Build history of the part. All positions in model axes, mm. Face numbers are marked on the shaded views. Give positions to 0.01 mm unless a question says otherwise; leave off trailing zeros. Loops run counter-clockwise (first coordinate to the right, second up) from the corner with the lowest first, then second, coordinate; pieces in that order, holes last. Notation, with made-up numbers: (61, 71) - (86, 71) arc R14 ccw to (86, 76) - close; hole circle Ø9 at (72.25, 2). An arc over 180 degrees is marked (long way). Return JSON: item names as keys, results as strings. Group by question number.
1) Slice it at D-D (y = 20.75). List the corners of the cut face in (x, z), and give its area (3 significant figures).
2) Drop flat-ended pins along their axis: pin 1 (4 mm diameter, centred on x = 34, z = 0, fed in from +Y); pin 2 (10 mm diameter, centred on x = -30, y = 6.5, fed in from -Z); pin 3 (3 mm diameter, centred on x = 15.5, y = 24, fed in from +Z); pin 4 (18 mm diameter, centred on x = 0, z = 0, fed in from +Y). Give the stop position or say it passes through.
3) Slice it at A-A (x = 0). List the corners of the cut face in (y, z), and give its area (3 significant figures).
4) Drill centre lines: probe 1 along X at (y, z) = (14, 0); probe 2 along Z at (x, y) = (1, 19.5); probe 3 along X at (y, z) = (14, -36.5). Where is each one in solid material? Low to high. Write a range as from..to.
5) Mould opens along X. For the marked faces 1, 2 and 3 say: released by +X, released by -X, zero draft, split by the parting line, or undercut.
6) Slice it at B-B (z = 0). List the corners of the cut face in (x, y).
7) Slice it at C-C (y = 3.75). List the corners of the cut face in (x, z), and give its area (3 significant figures).
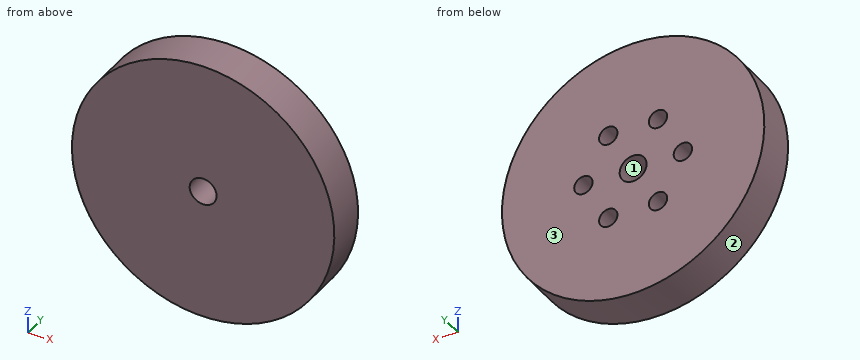
```python
from build123d import *

# Parameters (mm, degrees)
SKETCH1_R             = 97.5
BOSS_EXTRUDE1_DEPTH   = 30
SKETCH2_R             = 10
CUT_EXTRUDE1_DEPTH    = 142.111657917
SKETCH3_R             = 6.819096127
CUT_EXTRUDE2_DEPTH    = 20.141211
CIRPATTERN1_START     = 9.858789147
CIRPATTERN1_OUTLINE_R = 6.819096127
CIRPATTERN1_DEPTH     = 20.141210853


# Read off the part's stored shape, not the designer's step: CirPattern1
with BuildPart() as part:
    # Sketch1 → Boss-Extrude1 (new body)
    with BuildSketch(Plane(origin=(0, 0, 0), x_dir=(1, 0, 0), z_dir=(0, 1, 0))):
        with Locations(Location((0, 0, 0), (0, 0, 270))):
            Circle(SKETCH1_R)
    extrude(amount=BOSS_EXTRUDE1_DEPTH)

    # Sketch2 → Cut-Extrude1 (cut, through all)
    with BuildSketch(Plane(origin=(0, 0, 0), x_dir=(1, 0, 0), z_dir=(0, 1, 0))):
        with Locations(Location((0, 0, 0), (0, 0, 270))):
            Circle(SKETCH2_R)
    extrude(amount=CUT_EXTRUDE1_DEPTH, mode=Mode.SUBTRACT)

    # Sketch3 → Cut-Extrude2 (cut)
    with BuildSketch(Plane(origin=(0, 30, 0), x_dir=(1, 0, 0), z_dir=(0, 1, 0))):
        with Locations(Location((-36.967875527, 0, 0), (0, 0, 270))):
            Circle(SKETCH3_R)
    extrude(amount=-CUT_EXTRUDE2_DEPTH, mode=Mode.SUBTRACT)

    # CirPattern1 outline → CirPattern1 (cut)
    with BuildSketch(Plane(origin=(0, 0, 0), x_dir=(1, 0, 0), z_dir=(0, 1, 0)).offset(CIRPATTERN1_START)):
        with Locations((-18.483937763, -32.01511933)):
            Circle(CIRPATTERN1_OUTLINE_R)
        with Locations((18.483937763, -32.01511933)):
            Circle(CIRPATTERN1_OUTLINE_R)
        with Locations((36.967875527, 0)):
            Circle(CIRPATTERN1_OUTLINE_R)
        with Locations((18.483937763, 32.01511933)):
            Circle(CIRPATTERN1_OUTLINE_R)
        with Locations((-18.483937763, 32.01511933)):
            Circle(CIRPATTERN1_OUTLINE_R)
    extrude(amount=CIRPATTERN1_DEPTH, mode=Mode.SUBTRACT)


solid = part.part
```
Results:
{
 "1": {"outline": "circle Ø195 at (0, 0); hole circle Ø13.64 at (-36.97, 0); hole circle Ø13.64 at (-18.48, -32.02); hole circle Ø13.64 at (-18.48, 32.02); hole circle Ø20 at (0, 0); hole circle Ø13.64 at (18.48, -32.02); hole circle Ø13.64 at (18.48, 32.02); hole circle Ø13.64 at (36.97, 0)", "area": "28,700 mm2"},
 "2": {"pin 1": "y = 9.86", "pin 2": "z = -94.24", "pin 3": "z = 96.49", "pin 4": "through"},
 "3": {"outline": "(0, -97.5) - (30, -97.5) - (30, -10) - (0, -10) - close; (0, 10) - (30, 10) - (30, 97.5) - (0, 97.5) - close", "area": "5,250 mm2"},
 "4": {"probe 1": "-97.5..-43.79, -30.15..-10, 10..30.15, 43.79..97.5", "probe 2": "-97.49..-9.95, 9.95..97.49", "probe 3": "-90.41..-23.62, -13.35..13.35, 23.62..90.41"},
 "5": {"face 1": "undercut", "face 2": "split by the parting line", "face 3": "zero draft"},
 "6": {"outline": "(-97.5, 0) - (-10, 0) - (-10, 30) - (-30.15, 30) - (-30.15, 9.86) - (-43.79, 9.86) - (-43.79, 30) - (-97.5, 30) - close; (10, 0) - (97.5, 0) - (97.5, 30) - (43.79, 30) - (43.79, 9.86) - (30.15, 9.86) - (30.15, 30) - (10, 30) - close"},
 "7": {"outline": "circle Ø195 at (0, 0); hole circle Ø20 at (0, 0)", "area": "29,600 mm2"}
}
